```python
from build123d import *

# Parameters (mm, degrees)
SKETCH1_R           = 0.635
BOSS_EXTRUDE1_DEPTH = 0.889


with BuildPart() as part:
    # Sketch1 → Boss-Extrude1 (new body)
    with BuildSketch(Plane.XY):
        with BuildLine():
            Line((-3.698228745, 6.615080486), (-3.574085754, 7.856510393))
            ThreePointArc((-3.574085754, 7.856510393), (-3.409477564, 8.182620391), (-3.068606861, 8.313962504))
            Line((-3.068606861, 8.313962504), (-0.77533342, 8.313962504))
            ThreePointArc((-0.77533342, 8.313962504), (-0.681168949, 8.27218018), (-0.648963697, 8.174325532))
            Line((-0.648963697, 8.174325532), (-0.851111104, 6.152851468))
            ThreePointArc((-0.851111104, 6.152851468), (-0.97722427, 5.865544883), (-1.248062797, 5.707127408))
            ThreePointArc((-1.248062797, 5.707127408), (0, -5.842), (1.248062797, 5.707127408))
            ThreePointArc((1.248062797, 5.707127408), (0.97722427, 5.865544883), (0.851111104, 6.152851468))
            Line((0.851111104, 6.152851468), (0.648963697, 8.174325532))
            ThreePointArc((0.648963697, 8.174325532), (0.681168949, 8.27218018), (0.77533342, 8.313962504))
            Line((0.77533342, 8.313962504), (3.068606861, 8.313962504))
            ThreePointArc((3.068606861, 8.313962504), (3.409477564, 8.182620391), (3.574085754, 7.856510393))
            Line((3.574085754, 7.856510393), (3.698228745, 6.615080486))
            ThreePointArc((3.698228745, 6.615080486), (3.978211686, 5.684290697), (4.587301311, 4.926814687))
            ThreePointArc((4.587301311, 4.926814687), (0, -7.62), (-4.587301311, 4.926814687))
            ThreePointArc((-4.587301311, 4.926814687), (-3.978211686, 5.684290697), (-3.698228745, 6.615080486))
        make_face()
        with Locations((-1.651, 7.043962504)):
            Circle(SKETCH1_R, mode=Mode.SUBTRACT)
        with Locations((1.651, 7.043962504)):
            Circle(SKETCH1_R, mode=Mode.SUBTRACT)
    extrude(amount=BOSS_EXTRUDE1_DEPTH)


solid = part.part
```
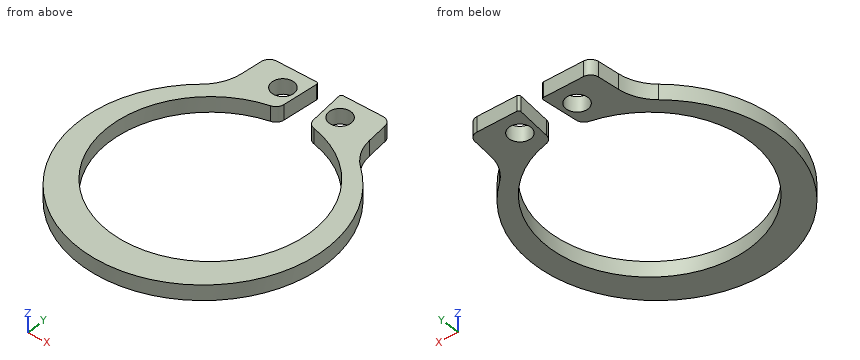
The listing builds one solid part. Answer for the finished solid, in the listing's coordinates (mm). Coordinates: 2 decimals unless noted, no trailing zeros. Loops run counter-clockwise (first coordinate to the right, second up) from the corner with the lowest first, then second, coordinate; pieces in that order, holes last. Notation, with made-up numbers: (68.5, 80.25) - (86.5, 80.25) arc R21 cw to (86.5, 115.25) - close; hole circle Ø1 at (-5.75, 61.25). An arc over 180 degrees is marked (long way). Use a Markdown table: item, result. Add a question column.
1) The part is cut by section A-A, the plane y = -1.25. Give the vertices of the cut face in (x, z).
2) Find the intervals of material crossed by line 1 (Y direction, x = -1.5, z = 0.8); line 2 (Y direction, x = 0, z = 0.35); line 3 (X direction, y = 0.75, z = 0.6), in increasing order.
3) The part is cut by section D-D, the plane y = 7.25. Give the vertices of the cut face in (x, z).
4) The part is cut by section B-B, the plane z = 0.65. Give the vertices of the cut face in (x, y) (3 decimals).
5) The part is cut by section C-C, the plane x = -2.5. Give the vertices of the cut face in (y, z), and give its area (3 significant figures).
Here are the results:
| question | item | result |
|---|---|---|
| 1 | outline | (-7.07, 0) - (-5.71, 0) - (-5.71, 0.89) - (-7.07, 0.89) - close; (5.71, 0) - (7.07, 0) - (7.07, 0.89) - (5.71, 0.89) - close |
| 2 | line 1 | y = -7.46 to -5.65, 5.65 to 6.43, 7.66 to 8.31 |
| 2 | line 2 | y = -7.62 to -5.84 |
| 2 | line 3 | x = -7 to -5.79, 5.79 to 7 |
| 3 | outline | (-3.63, 0) - (-2.25, 0) - (-2.25, 0.89) - (-3.63, 0.89) - close; (-1.05, 0) - (-0.74, 0) - (-0.74, 0.89) - (-1.05, 0.89) - close; (0.74, 0) - (1.05, 0) - (1.05, 0.89) - (0.74, 0.89) - close; (2.25, 0) - (3.63, 0) - (3.63, 0.89) - (2.25, 0.89) - close |
| 4 | outline | (-4.587, 4.927) arc R7.112 ccw (long way) to (4.587, 4.927) arc R2.54 cw to (3.698, 6.615) - (3.574, 7.857) arc R0.508 ccw to (3.069, 8.314) - (0.775, 8.314) arc R0.127 ccw to (0.649, 8.174) - (0.851, 6.153) arc R0.508 ccw to (1.248, 5.707) arc R5.842 cw (long way) to (-1.248, 5.707) arc R0.508 ccw to (-0.851, 6.153) - (-0.649, 8.174) arc R0.127 ccw to (-0.775, 8.314) - (-3.069, 8.314) arc R0.508 ccw to (-3.574, 7.857) - (-3.698, 6.615) arc R2.54 cw to start; hole circle Ø1.27 at (-1.651, 7.044); hole circle Ø1.27 at (1.651, 7.044) |
| 5 | outline | (-7.17, 0) - (-5.28, 0) - (-5.28, 0.89) - (-7.17, 0.89) - close; (5.28, 0) - (8.31, 0) - (8.31, 0.89) - (5.28, 0.89) - close |
| 5 | area | 4.37 mm^2 |
